```python
from build123d import *

# Parameters (mm, degrees)
F1_DEPTH = 25


with BuildPart() as f1:
    # F0 (on Top) → F1 (new body)
    with BuildSketch(Plane.XY):
        with BuildLine():
            Line((-31.411291, 67.580059), (-81.411291, 67.580059))
            Line((-81.411291, 67.580059), (-81.411291, 42.580059))
            Line((-81.411291, 42.580059), (-81.411291, -6.443731))
            Line((-81.411291, -6.443731), (-81.411291, -12.419941))
            Line((-81.411291, -12.419941), (-81.411291, -32.419941))
            Line((-81.411291, -32.419941), (-56.411291, -32.419941))
            Line((-56.411291, -32.419941), (-31.411291, -32.419941))
            Line((-31.411291, -32.419941), (-26.411291, -32.419941))
            Line((-26.411291, -32.419941), (28.588709, -32.419941))
            Line((28.588709, -32.419941), (53.588709, -32.419941))
            Line((53.588709, -32.419941), (78.588709, -32.419941))
            Line((78.588709, -32.419941), (78.588709, 42.580059))
            Line((78.588709, 42.580059), (78.588709, 67.580059))
            Line((78.588709, 67.580059), (28.588709, 67.580059))
            Line((28.588709, 67.580059), (28.588709, 37.580059))
            ThreePointArc((28.588709, 37.580059), (22.730845, 23.437924), (8.588709, 17.580059))
            Line((8.588709, 17.580059), (-11.411291, 17.580059))
            ThreePointArc((-11.411291, 17.580059), (-25.553426, 23.437924), (-31.411291, 37.580059))
            Line((-31.411291, 37.580059), (-31.411291, 67.580059))
        make_face()
        Polygon((-70.267661, -12.45164), (-70.249456, -12.419941), (-66.817294, -6.44373), (-63.366928, -0.435822), (-56.438742, -0.419972), (-49.510558, -0.404123), (-46.032739, -6.396182), (-42.554921, -12.388242), (-46.005287, -18.396151), (-49.455654, -24.40406), (-56.383839, -24.419909), (-63.312024, -24.435759), (-66.789843, -18.443699), align=None, mode=Mode.SUBTRACT)
        with BuildLine():
            ThreePointArc((-26.411291, -17.607526), (-31.411291, -12.607526), (-26.411291, -7.607526))
            Line((-26.411291, -7.607526), (23.588709, -7.607526))
            ThreePointArc((23.588709, -7.607526), (28.588709, -12.607526), (23.588709, -17.607526))
            Line((23.588709, -17.607526), (-26.411291, -17.607526))
        make_face(mode=Mode.SUBTRACT)
        Polygon((53.818598, -24.880686), (53.588709, -24.884927), (46.624383, -25.013412), (42.912332, -18.849403), (39.20028, -12.685393), (42.682443, -6.388658), (46.164606, -0.091922), (53.358821, 0.040804), (53.588709, 0.045045), (60.553035, 0.17353), (64.265087, -5.990479), (67.977138, -12.154488), (67.83034, -12.419941), (64.494975, -18.451224), (61.012812, -24.74796), align=None, mode=Mode.SUBTRACT)
        Polygon((-66.925847, 36.796972), (-70.10659, 42.580059), (-70.264714, 42.867554), (-66.67687, 48.794388), (-63.089025, 54.721223), (-56.162314, 54.577476), (-49.235601, 54.433729), (-45.896734, 48.363146), (-42.557867, 42.292564), (-46.145712, 36.36573), (-49.733557, 30.438895), (-56.411291, 30.577475), (-56.660269, 30.582642), (-63.58698, 30.72639), align=None, mode=Mode.SUBTRACT)
        Polygon((64.083761, 48.398469), (67.309461, 42.580059), (67.443021, 42.339147), (63.875125, 36.400282), (60.30723, 30.461417), (53.588709, 30.578245), (53.380073, 30.581873), (46.452918, 30.702329), (43.093658, 36.761649), (39.734397, 42.820971), (43.302293, 48.759836), (46.870189, 54.698701), (53.797345, 54.578245), (60.724501, 54.457789), align=None, mode=Mode.SUBTRACT)
    extrude(amount=F1_DEPTH)


solid = f1.part
```
Here's how the part is built. I have some questions about the finished solid (model axes, mm). A direction names the side the tool comes from. Coordinates: 2 decimals unless noted, no trailing zeros. Loops run counter-clockwise (first coordinate to the right, second up) from the corner with the lowest first, then second, coordinate; pieces in that order, holes last. Notation, with made-up numbers: (40.5, -39.75) - (91.5, -39.75) arc R24 ccw to (91.5, -27.75) - close; hole circle Ø3 at (88.25, 22.25). An arc over 180 degrees is marked (long way). Return JSON: item names as keys, results as strings. Group by question number.
Item 1: If we section it at C-C on x = -52: Write out the boundary of the cut face in (y, z).
Item 2: I need wall thicknesses on line 1 (Y direction, x = 59, z = 17.5); line 2 (Y direction, x = 53.5, z = 7.5); line 3 (X direction, y = 55, z = 20). Which ranges of each line are inside material? Lowest first, please. Write a range as from..to.
Item 3: If we section it at B-B on y = 22.5: Write out the boundary of the cut face in (x, z), and give its area (3 significant figures).
Item 4: If we section it at A-A on x = -15: Write out the boundary of the cut face in (y, z).
Item 5: On a 3-axis mill with a long thin cutter (end or side, diameter ignored), from which of +Z, -Z, +X, -X, +Y, -Y can I reach the whole of each face in a straight line? I mean faces 4 (the face through (-31.411, 52, 12)), 5 (the face through (78.589, 17, 12)), 6 (the face through (-1, -17.608, 12)). Say none if no direction works.
Item 6: We'd pull the mould along X, two halves only. Please class faces 1 (the face through (-81.411, 18, 12)), 2 (the face through (-3, -32.42, 12)), 3 (the face through (-31.41, -12.72, 12.32)): +X half, -X half, draft (parallel to the pull), parting line (faces both ways), or undercut.
Item 7: Will these pins go through, and if not, where does the flat tip stop? P1, Ø6, axis at x = 23.5, z = 11, coming from the +Y side; P2, Ø10, axis at x = 10.5, z = 8.5, coming from the +Y side; P3, Ø12.5, axis at x = -3.5, z = 9, coming from the +Y side.
Item 8: If we section it at D-D on z = 21.75: State how many separate pieces and enclosed holes the cut face has, and give its area (3 significant figures).
Calculated:
{
 "1": {"outline": "(-32.42, 0) - (-24.41, 0) - (-24.41, 25) - (-32.42, 25) - close; (-0.41, 0) - (30.49, 0) - (30.49, 25) - (-0.41, 25) - close; (54.49, 0) - (67.58, 0) - (67.58, 25) - (54.49, 25) - close"},
 "2": {"line 1": "y = -32.42..-24.79, 0.14..30.48, 54.49..67.58", "line 2": "y = -32.42..-24.89, 0.04..30.58, 54.58..67.58", "line 3": "x = -81.41..-31.41, 28.59..78.59"},
 "3": {"outline": "(-81.41, 0) - (-24.55, 0) - (-24.55, 25) - (-81.41, 25) - close; (21.73, 0) - (78.59, 0) - (78.59, 25) - (21.73, 25) - close", "area": "2,840 mm^2"},
 "4": {"outline": "(-32.42, 0) - (-17.61, 0) - (-17.61, 25) - (-32.42, 25) - close; (-7.61, 0) - (17.9, 0) - (17.9, 25) - (-7.61, 25) - close"},
 "5": {"face 4": "+Z, -Z, +Y", "face 5": "+Z, -Z, +X, +Y, -Y", "face 6": "+Z, -Z"},
 "6": {"face 1": "-X half", "face 2": "draft", "face 3": "undercut"},
 "7": {"P1": "stops at y = 28.68", "P2": "stops at y = 18.81", "P3": "stops at y = 17.58"},
 "8": {"separate pieces": "1", "enclosed holes": "5", "area": "10,600 mm^2"}
}
